Study the drawing (mm; zero at the part's minimum x, y, z) and answer. A direction names the side the tool comes from. Give positions to 0.01 mm unless a question says otherwise; leave off trailing zeros. Write each loop counter-clockwise with the first axis right and the second up, starting at its lowest first coordinate (ties: lowest second). Pieces come first, ordered by that corner, then holes. Notation, with made-up numbers: (18, -8.5) - (48, -8.5) arc R10 ccw to (48, 1.5) - close; hole circle Ø11 at (20.5, 52). An arc over 180 degrees is marked (long way). Return JSON: item names as keys, results as strings.
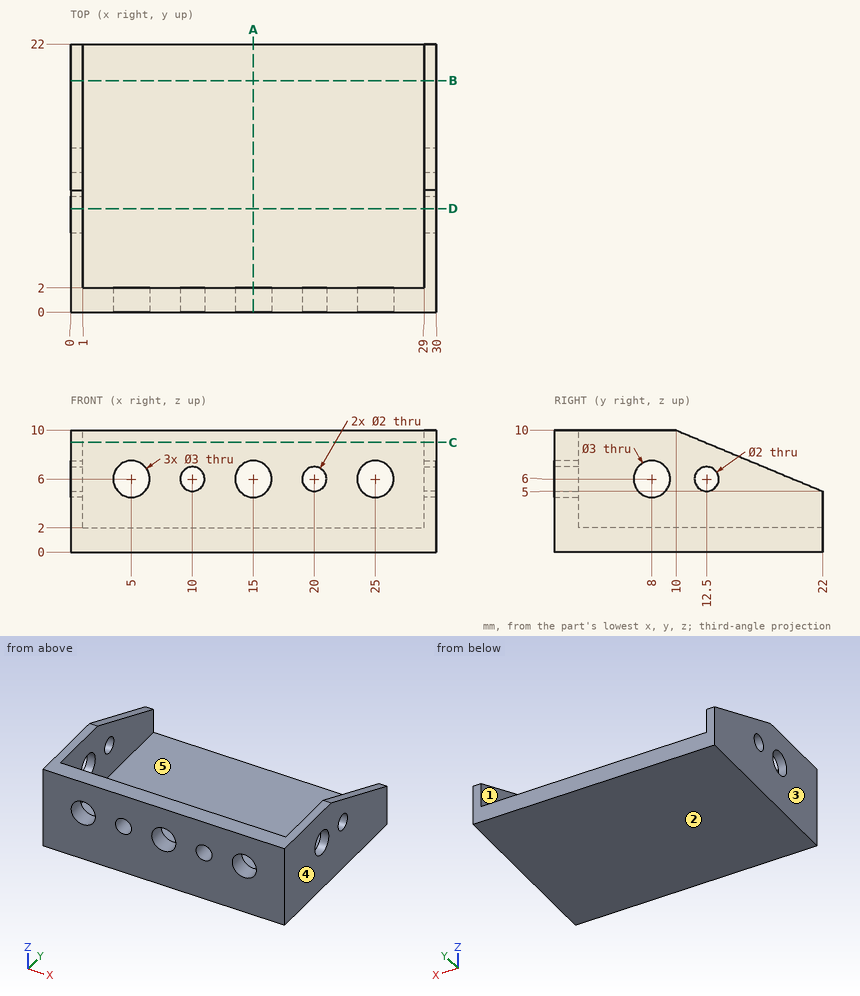
Item 1: For the marked faces 4 and 5, determine the directions among +Z, -Z, +X, -X, +Y, -Y from which every point of the face is accessible in a straight line to the end or side of a thin tool.
Answer below:
{"face 4": "+Z, -Z, +X, +Y, -Y", "face 5": "+Z, +Y"}
Item 2: Flat-ended cylindrical pins translate along their axes: P1, Ø1.8, axis at x = 25, z = 6, coming from the +Y side; P2, Ø10, axis at x = 17, y = 13, coming from the +Z side. Find the tip coordinate at first contact, or state that the pin passes through.
Answer below:
{"P1": "passes through", "P2": "stops at z = 2"}
Item 3: The mould has two halves that part along X. Classify the marked faces 1, 2 and 3: +X half, -X half, draft (parallel to the pull), parting line (faces both ways), or undercut.
Answer below:
{"face 1": "undercut", "face 2": "draft", "face 3": "-X half"}
Item 4: A cutting plane is placed at A-A on x = 15. Determine the outline of the cut face in (y, z).
Answer below:
{"outline": "(0, 0) - (22, 0) - (22, 2) - (2, 2) - (2, 4.5) - (0, 4.5) - close; (0, 7.5) - (2, 7.5) - (2, 10) - (0, 10) - close"}
Item 5: A cutting plane is placed at C-C on z = 9. Determine the outline of the cut face in (x, y), then the cut area to 3 significant figures.
Answer below:
{"outline": "(0, 0) - (30, 0) - (30, 12.4) - (29, 12.4) - (29, 2) - (1, 2) - (1, 12.4) - (0, 12.4) - close", "area": "80.8 mm²"}
Item 6: A cutting plane is placed at B-B on y = 19. Determine the outline of the cut face in (x, z), then the cut area to 3 significant figures.
Answer below:
{"outline": "(0, 0) - (30, 0) - (30, 6.25) - (29, 6.25) - (29, 2) - (1, 2) - (1, 6.25) - (0, 6.25) - close", "area": "68.5 mm²"}
Item 7: A cutting plane is placed at D-D on y = 8.5. Determine the outline of the cut face in (x, z).
Answer below:
{"outline": "(0, 0) - (30, 0) - (30, 4.59) - (29, 4.59) - (29, 2) - (1, 2) - (1, 4.59) - (0, 4.59) - close; (0, 7.41) - (1, 7.41) - (1, 10) - (0, 10) - close; (29, 7.41) - (30, 7.41) - (30, 10) - (29, 10) - close"}
Item 8: Consider L1, parallel to X at y = 1.4, z = 6; L2, parallel to X at y = 20.5, z = 4.5; L3, parallel to Y at x = 0.4, z = 6. Determine where each line is inside the solid, lowest interval first.
Answer below:
{"L1": "x = 0 to 3.5, 6.5 to 9, 11 to 13.5, 16.5 to 19, 21 to 23.5, 26.5 to 30", "L2": "x = 0 to 1, 29 to 30", "L3": "y = 0 to 6.5, 9.5 to 11.5, 13.5 to 19.6"}
